```python
from build123d import *

# Parameters (mm, degrees)
F2_T       = -2.5
F3_R       = 2
F4_SIZE2   = 1
F4_SIZE    = 2
F4_2_SIZE2 = 1
F4_2_SIZE  = 2


with BuildPart() as f1:
    # F0 (on Front) → F1 (revolve)
    with BuildSketch(Plane.XZ):
        Polygon((0, 0), (0, 44), (-7, 44), (-7, 29), (-16, 20), (-16, 0), align=None)
    revolve(axis=Axis((0, 0, 22), (0, 0, 1)))

    # F2
    f2_openings = [f1.faces().sort_by_distance(p)[0] for p in [
        (0, 0, 44),
        (0, 0, 0),
    ]]
    offset(amount=F2_T, openings=f2_openings, kind=Kind.INTERSECTION)

    # F3
    f3_edges = [f1.edges().sort_by_distance(p)[0] for p in [
        (7, 0, 29),
        (13.5, 0, 18.964466),
    ]]
    fillet(f3_edges, radius=F3_R)

    # F4
    f4_edges = [f1.edges().sort_by_distance(p)[0] for p in [
        (16, 0, 0),
    ]]
    f4_side = f1.faces().sort_by_distance((16, 0, 10))[0]
    chamfer(f4_edges, length=F4_SIZE, length2=F4_SIZE2, reference=f4_side)

    # F4#2
    f4_2_edges = [f1.edges().sort_by_distance(p)[0] for p in [
        (4.5, 0, 44),
    ]]
    f4_2_side = f1.faces().sort_by_distance((4.5, 0, 35.982233))[0]
    chamfer(f4_2_edges, length=F4_2_SIZE, length2=F4_2_SIZE2, reference=f4_2_side)


solid = f1.part
```
Work out the finished part from the listing and answer in its coordinate system (mm). Coordinates: 2 decimals unless noted, no trailing zeros. Write each loop counter-clockwise with the first axis right and the second up, starting at its lowest first coordinate (ties: lowest second). Pieces come first, ordered by that corner, then holes. Notation, with made-up numbers: (42.5, -9.5) - (97.5, -9.5) arc R31 cw to (97.5, 23.5) - close; hole circle Ø7 at (68, 13.5). An arc over 180 degrees is marked (long way). Answer as a JSON object with one key per item and string values.
Q1. Find section A-A (z = 38.5). Write down the section's boundary in (x, y), plus the area to 3 significant figures.
Results list:
{"outline": "circle Ø14 at (0, 0); hole circle Ø9 at (0, 0)", "area": "90.3 mm^2"}
Q2. Consider L1, parallel to Y at x = 0, z = 37; L2, parallel to X at y = 0, z = 12. Determine where each line is inside the solid, lowest interval first. Write a range as from..to.
Results list:
{"L1": "y = -7..-4.5, 4.5..7", "L2": "x = -16..-13.5, 13.5..16"}
Q3. Find section B-B (z = 10). Write down the section's boundary in (x, y).
Results list:
{"outline": "circle Ø32 at (0, 0); hole circle Ø27 at (0, 0)"}
Q4. Given pin 1 Ø6 at (x, z) = (5.5, 10.5) entering from +Y; pin 2 Ø4 at (y, z) = (-2.5, 7.5) entering from -X; pin 3 Ø2 at (x, y) = (8, 5.5) entering from -Z, each flat-ended and moving along its own axis, determine where each tip first touches the part or whether it passes through.
Results list:
{"pin 1": "stops at y = 15.8", "pin 2": "stops at x = -15.99", "pin 3": "stops at z = 21.76"}
Q5. For a pull along X with two mould halves and no side action, classify faces 1 (the flat face through (-4, 4, 44)), 2 (the cylindrical face through (-3.763, -5.902, 36.815)), 3 (the cylindrical face through (2.93, 13.18, 8.94)) as pulls with the +X half, pulls with the -X half, needs draft (parallel to the pull), parting line crosses it, or undercut.
Results list:
{"face 1": "needs draft", "face 2": "parting line crosses it", "face 3": "undercut"}
